Here's how the part is built. I have some questions about the finished solid (model axes, mm). A direction names the side the tool comes from. Round coordinates to 2 decimals unless told otherwise and drop trailing zeros. Order: outer loops, then holes, each group sorted by start corner. A loop starts at its lowest first (then second) coordinate and runs counter-clockwise, first axis right, second up. Notation, with made-up numbers: (-8, 55.5) -> (15, 55.5) arc R26 ccw to (15, 80.5) -> close; hole circle Ø7 at (-3, -21). An arc over 180 degrees is marked (long way). Answer in a Markdown table with one row per item.
```python
from build123d import *

# Parameters (mm, degrees)
SKETCH001_W  = 0.5
SKETCH001_H  = 2
POCKET_DEPTH = 2.5


with BuildPart() as part:
    # Sketch → Revolution (revolve)
    with BuildSketch(Plane.YZ):
        Polygon((0, 0), (-1, 0), (-1, -3), (-0.8, -3), (-0.8, -9), (-0.7, -9), (-0.7, -11), (0, -11), align=None)
    revolve(axis=Axis((0, 0, 0), (0, 0, 1)))

    # Sketch001 (on Face1 of Revolution) → Pocket (cut)
    with BuildSketch(Plane(origin=(0, 0, 0), x_dir=(0, -1, 0), z_dir=(0, 0, 1))):
        Rectangle(SKETCH001_W, SKETCH001_H)
    extrude(amount=-POCKET_DEPTH, mode=Mode.SUBTRACT)


solid = part.part
```
1. Suppose I cut it at A-A on z = -1.25. Write out the boundary of the cut face in (x, y), then the cut area to 3 significant figures.
Numbers:
| item | result |
|---|---|
| outline | (-0.97, -0.25) arc R1 ccw to (0.97, -0.25) -> close; (-0.97, 0.25) -> (0.97, 0.25) arc R1 ccw to start |
| area | 2.15 mm2 |
2. Suppose I cut it at C-C on y = 0. Write out the boundary of the cut face in (x, z), then the cut area to 3 significant figures.
Numbers:
| item | result |
|---|---|
| outline | (-1, -3) -> (-0.8, -3) -> (-0.8, -9) -> (-0.7, -9) -> (-0.7, -11) -> (0.7, -11) -> (0.7, -9) -> (0.8, -9) -> (0.8, -3) -> (1, -3) -> (1, -2.5) -> (-1, -2.5) -> close |
| area | 13.4 mm2 |
3. We'd pull the mould along Y, two halves only. Please class faces 4 (the face through (0, 0.25, -1)), 5 (the face through (-0.49, 0.63, -6.04)), 6 (the face through (0, 0, -11)): released by +Y, released by -Y, zero draft, split by the parting line, or undercut.
Numbers:
| item | result |
|---|---|
| face 4 | undercut |
| face 5 | split by the parting line |
| face 6 | zero draft |
4. Please list where these lines run through material, in increasing order: line 1 along Z through (x, y) = (-0.1, 0.75); line 2 along Y through (x, z) = (0.4, -0.5); line 3 along Z through (x, y) = (-0.1, 0.1).
Numbers:
| item | result |
|---|---|
| line 1 | z = -9 to 0 |
| line 2 | y = -0.92 to -0.25, 0.25 to 0.92 |
| line 3 | z = -11 to -2.5 |
5. Suppose I cut it at B-B on x = 0. Write out the boundary of the cut face in (y, z).
Numbers:
| item | result |
|---|---|
| outline | (-1, -3) -> (-0.8, -3) -> (-0.8, -9) -> (-0.7, -9) -> (-0.7, -11) -> (0.7, -11) -> (0.7, -9) -> (0.8, -9) -> (0.8, -3) -> (1, -3) -> (1, 0) -> (0.25, 0) -> (0.25, -2.5) -> (-0.25, -2.5) -> (-0.25, 0) -> (-1, 0) -> close |
6. For faces 1 (the face through (0, 0.7, -10)), 2 (the face through (0, -0.25, -1)), 3 (the face through (0, -1, -2)), which set-ups out of +Z, -Z, +X, -X, +Y, -Y let a thin tool reach every point of the face, with its end or its side?
Numbers:
| item | result |
|---|---|
| face 1 | -Z |
| face 2 | +Z, +X, -X |
| face 3 | +Z, -Z |
7. Suppose I cut it at D-D on z = -6.25. Write out the boundary of the cut face in (x, y).
Numbers:
| item | result |
|---|---|
| outline | circle Ø1.6 at (0, 0) |
